Source: three-view drawing plus pictorial views. Frame: mm from the lowest corner of the part. Coordinates: 2 decimals unless noted, no trailing zeros. Write each loop counter-clockwise with the first axis right and the second up, starting at its lowest first coordinate (ties: lowest second). Pieces come first, ordered by that corner, then holes. Notation, with made-up numbers: (78, 51.5) - (122, 51.5) arc R14 ccw to (122, 66.5) - close; hole circle Ø2 at (30.5, 40.25). An arc over 180 degrees is marked (long way). Put each result on its own line as item: value. Start each with the question number.
1. Cut plane C-C, the plane z = 33. Return loops of the section in (x, y), and give its area (3 significant figures).
2. Pin query (flat end, axial travel): pin 1 (1 mm diameter, centred on y = 0.5, z = 23.5, fed in from -X) (1 decimal); pin 2 (0.9 mm diameter, centred on x = 12, y = 1.5, fed in from -Z). Return the tip coordinate at first contact, or that it passes through.
3. Cut plane B-B, the plane x = 14. Return loops of the section in (y, z) (1 decimal).
4. Line query: line 1 (X direction, y = 1, z = 8.5) (1 decimal); line 2 (Z direction, x = 26.5, y = 2.1); line 3 (X direction, y = 0.55, z = 21.5) (1 decimal). Output: solid intervals per line, ascending.
5. Cut plane A-A, the plane y = 1.95. Return loops of the section in (x, z) (1 decimal).
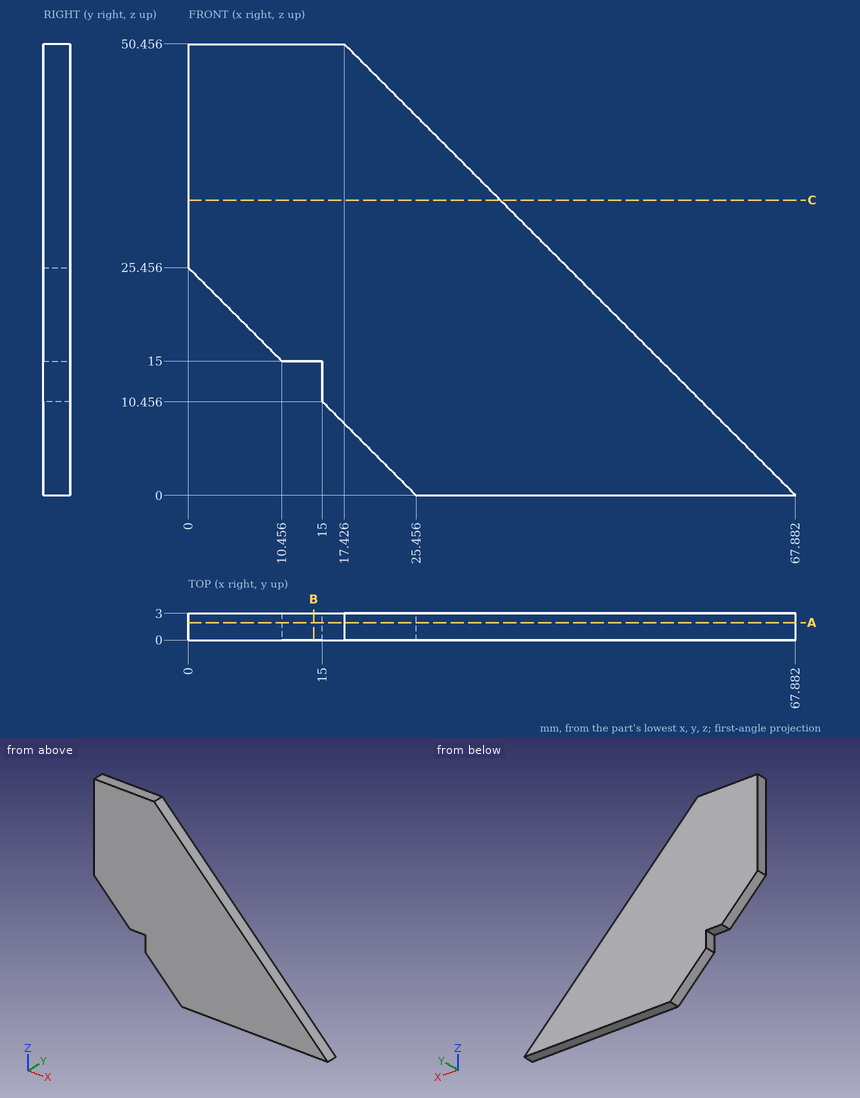
Report:
1. outline: (0, 0) - (34.88, 0) - (34.88, 3) - (0, 3) - close
1. area: 105 mm^2
2. pin 1: stops at x = 1.5
2. pin 2: stops at z = 15
3. outline: (0, 15) - (3, 15) - (3, 50.5) - (0, 50.5) - close
4. line 1: x = 17 to 59.4
4. line 2: z = 0 to 41.38
4. line 3: x = 4 to 46.4
5. outline: (0, 25.5) - (10.5, 15) - (15, 15) - (15, 10.5) - (25.5, 0) - (67.9, 0) - (17.4, 50.5) - (0, 50.5) - close
